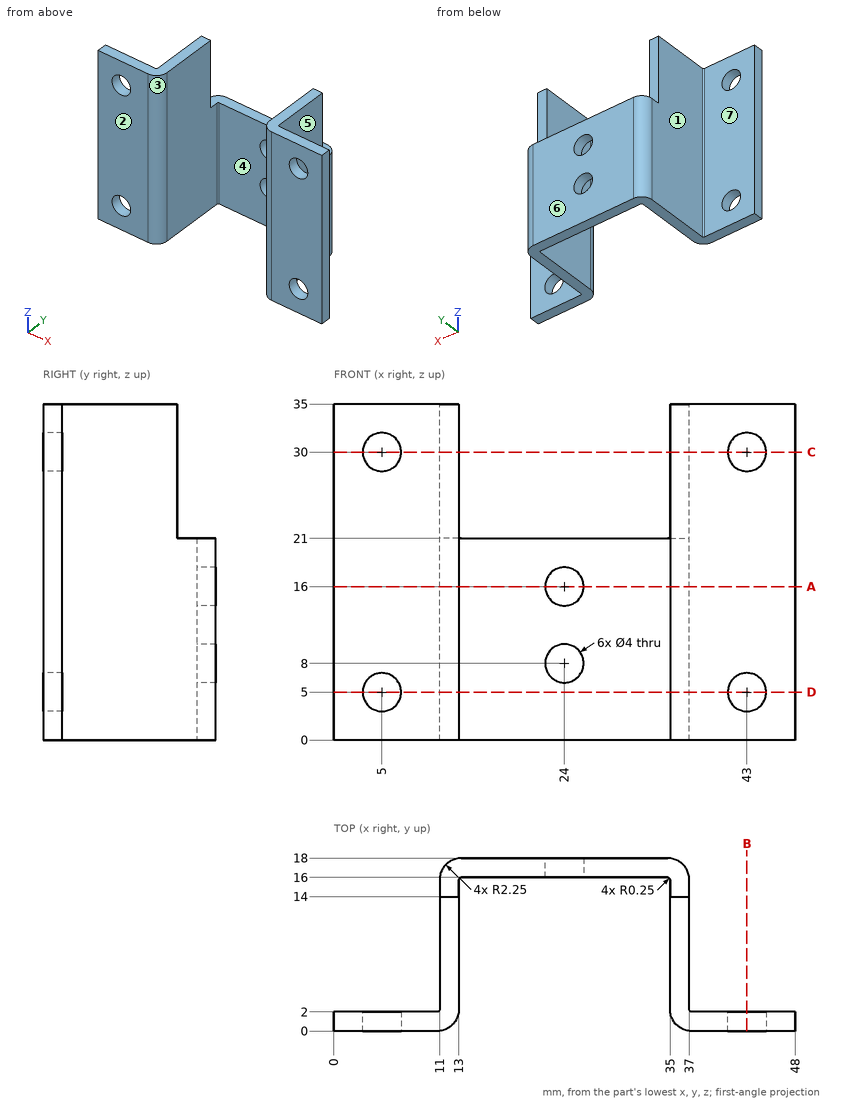
Geometry check sheet. Reference: drawing and pictorial views, mm from the part's lowest x, y, z. A direction names the side the tool comes from. Coordinates: 2 decimals unless noted, no trailing zeros. Loops run counter-clockwise (first coordinate to the right, second up) from the corner with the lowest first, then second, coordinate; pieces in that order, holes last. Notation, with made-up numbers: (63.25, -11) - (69.25, -11) arc R23 cw to (69.25, 10) - close; hole circle Ø7 at (26, 6). An arc over 180 degrees is marked (long way). Return JSON: item names as keys, results as strings.
1. Mould release check, pull along X, two halves, no side actions. Record for the marked faces 1, 2 and 3: +X half, -X half, draft (parallel to the pull), parting line (faces both ways), or undercut.
Established:
{"face 1": "-X half", "face 2": "draft", "face 3": "undercut"}
2. Go/stop test with flat-tipped pins: pin 1 (3 mm diameter, centred on x = 4, z = 23.5, fed in from +Y); pin 2 (1.6 mm diameter, centred on x = 36, z = 29, fed in from +Y); pin 3 (1.5 mm diameter, centred on x = 33.5, z = 20.5, fed in from -Y). Record where each tip stops, or that it passes through.
Established:
{"pin 1": "stops at y = 2", "pin 2": "stops at y = 14", "pin 3": "stops at y = 16"}
3. Section check C-C, the plane z = 30. Record the boundary of the cut face in (x, y), then the cut area to 3 significant figures.
Established:
{"outline": "(0, 0) - (3, 0) - (3, 2) - (0, 2) - close; (7, 0) - (10.75, 0) arc R2.25 ccw to (13, 2.25) - (13, 14) - (11, 14) - (11, 2.25) arc R0.25 cw to (10.75, 2) - (7, 2) - close; (35, 2.25) arc R2.25 ccw to (37.25, 0) - (41, 0) - (41, 2) - (37.25, 2) arc R0.25 cw to (37, 2.25) - (37, 14) - (35, 14) - close; (45, 0) - (48, 0) - (48, 2) - (45, 2) - close", "area": "81.9 mm2"}
4. Tool access check on the marked faces 4, 5, 6 and 7. Record the directions out of +Z, -Z, +X, -X, +Y, -Y that give a thin tool (end or side, any length) a straight path to the whole face; none if there is none.
Established:
{"face 4": "+Z, -Z, -Y", "face 5": "+Z, -Z, +X, +Y", "face 6": "+Z, -Z, +X, -X, +Y", "face 7": "+Z, -Z, -X, +Y"}
5. Section check D-D, the plane z = 5. Record the boundary of the cut face in (x, y).
Established:
{"outline": "(0, 0) - (3, 0) - (3, 2) - (0, 2) - close; (7, 0) - (10.75, 0) arc R2.25 ccw to (13, 2.25) - (13, 15.75) arc R0.25 cw to (13.25, 16) - (34.75, 16) arc R0.25 cw to (35, 15.75) - (35, 2.25) arc R2.25 ccw to (37.25, 0) - (41, 0) - (41, 2) - (37.25, 2) arc R0.25 cw to (37, 2.25) - (37, 15.75) arc R2.25 ccw to (34.75, 18) - (13.25, 18) arc R2.25 ccw to (11, 15.75) - (11, 2.25) arc R0.25 cw to (10.75, 2) - (7, 2) - close; (45, 0) - (48, 0) - (48, 2) - (45, 2) - close"}
6. Section check B-B, the plane x = 43. Record the boundary of the cut face in (y, z), then the cut area to 3 significant figures.
Established:
{"outline": "(0, 0) - (2, 0) - (2, 3) - (0, 3) - close; (0, 7) - (2, 7) - (2, 28) - (0, 28) - close; (0, 32) - (2, 32) - (2, 35) - (0, 35) - close", "area": "54.0 mm2"}
7. Section check A-A, the plane z = 16. Record the boundary of the cut face in (x, y).
Established:
{"outline": "(0, 0) - (10.75, 0) arc R2.25 ccw to (13, 2.25) - (13, 15.75) arc R0.25 cw to (13.25, 16) - (22, 16) - (22, 18) - (13.25, 18) arc R2.25 ccw to (11, 15.75) - (11, 2.25) arc R0.25 cw to (10.75, 2) - (0, 2) - close; (26, 16) - (34.75, 16) arc R0.25 cw to (35, 15.75) - (35, 2.25) arc R2.25 ccw to (37.25, 0) - (48, 0) - (48, 2) - (37.25, 2) arc R0.25 cw to (37, 2.25) - (37, 15.75) arc R2.25 ccw to (34.75, 18) - (26, 18) - close"}
8. Thickness scan on L1, parallel to Z at x = 43, y = 1.2; L2, parallel to Z at x = 24, y = 17.2; L3, parallel to X at y = 15, z = 9. Record the ranges inside material, lowest first.
Established:
{"L1": "z = 0 to 3, 7 to 28, 32 to 35", "L2": "z = 0 to 6, 10 to 14, 18 to 21", "L3": "x = 11 to 13, 35 to 37"}
